Autodesk Inventor part; units mm, degrees
ref_plane "YZ Plane" through (0, 0, 0) normal (1, 0, 0) x (0, 1, 0)
ref_plane "XZ Plane" through (0, 0, 0) normal (0, 1, 0) x (-1, 0, 0)
ref_plane "XY Plane" through (0, 0, 0) normal (0, 0, 1) x (1, 0, 0)
sketch "Sketch1" plane through (0, 0, 0) normal (1, 0, 0) x (0, 1, 0)
  line L0 (0, 66) -> (0, 0)
  line L1 (-57.5, 0) -> (326.5, 0) construction
  line L2 (102.5, 12) -> (0, 12)
  circle A0 centre (6.5, 5) radius 1.5
  circle A1 centre (22.5, 5) radius 1.5
  circle A2 centre (38.5, 5) radius 1.5
  circle A3 centre (54.5, 5) radius 1.5
  circle A4 centre (70.5, 5) radius 1.5
  circle A5 centre (86.5, 5) radius 1.5
  line L3 (0, 0) -> (102.5, 0)
  line L4 (102.5, 0) -> (102.5, 12)
  line L5 (102.5, 66) -> (0, 66) construction
  line L6 (0, 66) -> (0, 0)
  line L7 (102.5, 12) -> (102.5, 66) construction
  line L8 (102.5, 12) -> (0, 66)
  line L9 (8, 0) -> (8, 61.7854)
  point P0 (8, 12)
  dimension "d0" = 12
  dimension "d1" = 3
  dimension "d2" = 5
  dimension "d3" = 6.5
  dimension "d6" = 16
  dimension "d11" = 16
  dimension "d12" = 66
  dimension "d19" = 8
extrude "Extrusion1" add sketch "Sketch1" along normal blind 10 contours L8 L9 L2 L0 | A0 | L2 L9 L3 L0 | L8 L2 L9 | L2 L4 L3 L9 | A2 | A4
extrude "Extrusion2" add sketch "Sketch1" along normal blind 22.5 from surface at 10 contours L8 L9 L2 L0 | A0 | L2 L9 L3 L0 | L2 L4 L3 L9 | A2 | A4
extrude "Extrusion3" add sketch "Sketch1" along normal blind 10 from surface at 32.5 contours L8 L9 L2 L0 | A0 | L2 L9 L3 L0 | L8 L2 L9 | L2 L4 L3 L9 | A2 | A4
sketch "Sketch2" plane through (10, 8, 61.7854) normal (0, 1, 0) x (1, 0, 0)
  line L0 (22.5, 0) -> (22.5, 49.7854)
  line L1 (0, 49.7854) -> (22.5, 49.7854)
  line L2 (0, 0) -> (0, 49.7854)
  line L3 (0, 0) -> (22.5, 0)
  circle A0 centre (11.25, 40.8927) radius 2.8
  circle A1 centre (11.25, 8.8927) radius 2.8
  line L4 (0, 49.7854) -> (22.5, 49.7854) construction
  line L5 (11.25, 49.7854) -> (11.25, 0) construction
  line L6 (0, 0) -> (22.5, 0) construction
  point P0 (-10, 61.7854)
  dimension "d20" = 5.6
  dimension "d21" = 8.8927
  dimension "d22" = 49.7854
  dimension "d23" = 32
extrude "Extrusion4" cut sketch "Sketch2" against normal blind 22.5 contours A0 | A1
sketch "Sketch3" plane through (10, 8, 12) normal (0, 0, 1) x (1, 0, 0)
  line L0 (11.1125, 41.275) -> (11.1125, 12.7) construction
  line L1 (0.74, 41.275) -> (0.74, 12.7)
  line L2 (21.485, 12.7) -> (21.485, 41.275)
  arc A0 (21.485, 41.275) -> (0.74, 41.275) centre (11.1125, 41.275) ccw
  arc A1 (0.74, 12.7) -> (21.485, 12.7) centre (11.1125, 12.7) ccw
  point P0 (-10, -8)
  point P1 (11.1125, 26.9875)
extrude "Extrusion5" cut sketch "Sketch3" against normal through all
equation "\"d21\" = -0.5 * d23 + 0.5 * d22"
properties part number "Slide Support"
Verification items for the finished model (mm, model axes). A direction names the side the tool comes from. Coordinates: 2 decimals unless noted, no trailing zeros. Write each loop counter-clockwise with the first axis right and the second up, starting at its lowest first coordinate (ties: lowest second). Pieces come first, ordered by that corner, then holes. Notation, with made-up numbers: M 46.5,46.25 L 98.5,46.25 A38 ccw 98.5,84.25 Z; hole C -13,87.5 d6. An arc over 180 degrees is marked long. Answer as a JSON object with one key per item and string values. Group by question number.
(1) Material ranges on line 1 (X direction, y = 12, z = 42); line 2 (X direction, y = 6, z = 53); line 3 (Z direction, x = 11, y = 15.5), recorded low to high.
(2) Cross-section at A-A, the plane z = 9. Record the cut outline in (x, y) (1 decimal), and give its area (3 significant figures).
(3) Gauge pin test, flat ends, axial feed: pin 1 (4 mm diameter, centred on y = 54.5, z = 5, fed in from +X); pin 2 (25 mm diameter, centred on x = 20, y = 40.5, fed in from +Z); pin 3 (6.5 mm diameter, centred on x = 21.25, z = 20.89, fed in from +Y); pin 4 (12 mm diameter, centred on x = 20.5, y = 62.5, fed in from +Z). Record the tip position at first contact, or that the pin passes through.
(4) Release check for a two-part mould opening along Z. For faces 4 (the face through (6.79, 51.97, 38.62)), 5 (the face through (7, 56, 5)), 6 (the face through (10, 34, 26)) record: +Z half, -Z half, draft (parallel to the pull), parting line (faces both ways), or undercut.
(5) Cross-section at B-B, the plane x = 21.25. Record the cut outline in (y, z), and give its area (3 significant figures).
(6) Cross-section at D-D, the plane x = 36. Record the cut outline in (y, z).
(7) Tool access check on faces 1 (the face through (10.74, 35, 6)), 2 (the face through (21, 8, 37)), 3 (the face through (21, 62, 0)). Record the directions out of +Z, -Z, +X, -X, +Y, -Y that give a thin tool (end or side, any length) a straight path to the whole face; none if there is none.
(8) Cross-section at C-C, the plane y = 86.5. Record the cut outline in (x, z), and give its area (3 significant figures).
Reply:
{
 "1": {"line 1": "0 to 10, 32.5 to 42.5", "line 2": "0 to 18.45, 24.05 to 42.5", "line 3": "0 to 12"},
 "2": {"outline": "M 0,0 L 42.5,0 L 42.5,102.5 L 0,102.5 Z; hole M 10.7,20.7 A10.4 ccw 31.5,20.7 L 31.5,49.3 A10.4 ccw 10.7,49.3 Z", "area": "3,430 mm²"},
 "3": {"pin 1": "x = 42.5", "pin 2": "z = 48.61", "pin 3": "y = 8", "pin 4": "z = 12"},
 "4": {"face 4": "+Z half", "face 5": "undercut", "face 6": "draft"},
 "5": {"outline": "M 0,0 L 10.33,0 L 10.33,12 L 8,12 L 8,18.09 L 0,18.09 Z; M 0,23.69 L 8,23.69 L 8,50.09 L 0,50.09 Z; M 0,55.69 L 8,55.69 L 8,61.79 L 0,66 Z; M 59.65,0 L 102.5,0 L 102.5,12 L 59.65,12 Z; hole C 86.5,5 d3", "area": "957 mm²"},
 "6": {"outline": "M 0,0 L 102.5,0 L 102.5,12 L 0,66 Z; hole C 22.5,5 d3; hole C 54.5,5 d3; hole C 86.5,5 d3"},
 "7": {"face 1": "+Z, -Z", "face 2": "+Z, +Y", "face 3": "-Z, +X, -X, +Y, -Y"},
 "8": {"outline": "M 0,0 L 42.5,0 L 42.5,3.5 L 0,3.5 Z; M 0,6.5 L 42.5,6.5 L 42.5,20.43 L 32.5,20.43 L 32.5,12 L 10,12 L 10,20.43 L 0,20.43 Z", "area": "551 mm²"}
}
